```python
from build123d import *

# Parameters (mm, degrees)
F0_R     = 3
F1_DEPTH = 6.35
F2_W     = 12.7
F2_H     = 6.35
F3_DEPTH = 6.35


with BuildPart() as f1:
    # F0 (on Front) → F1 (new body)
    with BuildSketch(Plane.XZ):
        with BuildLine():
            Line((63.5, 0), (12.220363, 181.257272))
            ThreePointArc((12.220363, 181.257272), (0, 190.5), (-12.220363, 181.257272))
            Line((-12.220363, 181.257272), (-63.5, 0))
            Line((-63.5, 0), (-44.45, 0))
            Line((-44.45, 0), (-30.078132, 50.8))
            Line((-30.078132, 50.8), (30.078132, 50.8))
            Line((30.078132, 50.8), (44.45, 0))
            Line((44.45, 0), (63.5, 0))
        make_face()
        Polygon((24.688682, 69.85), (-24.688682, 69.85), (-6.723847, 133.35), (6.723847, 133.35), align=None, mode=Mode.SUBTRACT)
        with Locations((0, 177.8)):
            Circle(F0_R, mode=Mode.SUBTRACT)
    extrude(amount=F1_DEPTH)

    # F2 (on face) → F3 (join)
    with BuildSketch(Plane(origin=(0, 0, 0), x_dir=(1, 0, 0), z_dir=(0, 0, -1))):
        with Locations((-50.8, 3.175)):
            Rectangle(F2_W, F2_H)
        with Locations((50.8, 3.175)):
            Rectangle(F2_W, F2_H)
    extrude(amount=F3_DEPTH)


solid = f1.part
```
CAD build for the part. Positions are in the model's coordinates, mm. A direction names the side the tool comes from. Coordinates: 2 decimals unless noted, no trailing zeros. Write each loop counter-clockwise with the first axis right and the second up, starting at its lowest first coordinate (ties: lowest second). Pieces come first, ordered by that corner, then holes.
(1) Cut at D-D, the plane z = 177.8. List the corners of the cut face in (x, y).
(2) 3-axis set-ups, long thin cutter, end or side, ignore diameter. For faces 1 (the face through (-37.365, -3.131, 25.044)), 2 (the face through (0, -3, 133.35)), 3 (the face through (-57.15, -3, -3)): which of +Z, -Z, +X, -X, +Y, -Y reach the whole face in a straight line?
(3) Cut at B-B, the plane z = 24.5. List the corners of the cut face in (x, y).
(4) Cut at C-C, the plane x = 0. List the corners of the cut face in (y, z).
(5) Two-plate mould, pull along X, no slides. Class faces 4 (the face through (44.45, -3, -3)), 5 (the face through (51, -3, -6.35)), 6 (the face through (-37.5, -3.1, 91.9)): +X half, -X half, draft (parallel to the pull), parting line (faces both ways), or undercut.
(6) Cut at A-A, the plane y = -3.75. List the corners of the cut face in (x, z), and give its area (3 significant figures).
(7) Flat gauge pins, fed straight in: pin 1 (3 mm diameter, centred on x = -2, y = -3, fed in from -Z); pin 2 (3 mm diameter, centred on x = -61.5, y = -2.5, fed in from -Z); pin 3 (3 mm diameter, centred on x = 9.5, y = -2, fed in from +Z). Where does each tip first touch, or does it go through?
(8) Drill centre lines: probe 1 along Z at (x, y) = (0, -4); probe 2 along X at (y, z) = (-4.25, 177.8); probe 3 along Z at (x, y) = (4.5, -3.5). Where is each one in solid material? Low to high.
Geometry says:
1. outline: (-13.2, -6.35) - (-3, -6.35) - (-3, 0) - (-13.2, 0) - close; (3, -6.35) - (13.2, -6.35) - (13.2, 0) - (3, 0) - close
2. face 1: -Z, +Y, -Y
2. face 2: +Y, -Y
2. face 3: -Z, -X, +Y, -Y
3. outline: (-56.57, -6.35) - (-37.52, -6.35) - (-37.52, 0) - (-56.57, 0) - close; (37.52, -6.35) - (56.57, -6.35) - (56.57, 0) - (37.52, 0) - close
4. outline: (-6.35, 50.8) - (0, 50.8) - (0, 69.85) - (-6.35, 69.85) - close; (-6.35, 133.35) - (0, 133.35) - (0, 174.8) - (-6.35, 174.8) - close; (-6.35, 180.8) - (0, 180.8) - (0, 190.5) - (-6.35, 190.5) - close
5. face 4: undercut
5. face 5: draft
5. face 6: -X half
6. outline: (-63.5, 0) - (-57.15, 0) - (-57.15, -6.35) - (-44.45, -6.35) - (-44.45, 0) - (-30.08, 50.8) - (30.08, 50.8) - (44.45, 0) - (44.45, -6.35) - (57.15, -6.35) - (57.15, 0) - (63.5, 0) - (12.22, 181.26) arc R12.7 ccw to (-12.22, 181.26) - close; hole (-24.69, 69.85) - (24.69, 69.85) - (6.72, 133.35) - (-6.72, 133.35) - close; hole circle Ø6 at (0, 177.8)
6. area: 8,240 mm2
7. pin 1: stops at z = 50.8
7. pin 2: stops at z = 0
7. pin 3: stops at z = 187.66
8. probe 1: z = 50.8 to 69.85, 133.35 to 174.8, 180.8 to 190.5
8. probe 2: x = -13.2 to -3, 3 to 13.2
8. probe 3: z = 50.8 to 69.85, 133.35 to 189.68
